Answer from the drawing. Dimensions are ordinates in mm from the lowest x, y and z of the part. A direction names the side the tool comes from. Round coordinates to 2 decimals unless told otherwise and drop trailing zeros. Order: outer loops, then holes, each group sorted by start corner. A loop starts at its lowest first (then second) coordinate and runs counter-clockwise, first axis right, second up. Notation, with made-up numbers: (31.25, 33) -> (35.25, 33) arc R17 cw to (35.25, 64) -> close; hole circle Ø5 at (41, -38). An arc over 180 degrees is marked (long way). Use a Markdown table: item, result. Add a question column.
1. Section C-C, the plane x = 6 is taken. Give the vertices of the cut face in (y, z).
2. Section D-D, the plane y = 13 is taken. Give the vertices of the cut face in (x, z).
3. Section B-B, the plane y = 22 is taken. Give the vertices of the cut face in (x, z).
4. Given pin 1 (12 mm diameter, centred on x = 29.5, y = 14.5, fed in from +Z); pin 2 (9 mm diameter, centred on x = 30, y = 22, fed in from +Z); pin 3 (1.5 mm diameter, centred on x = 34, z = 25.5, fed in from +Y), each flat-ended and moving along its own axis, determine where each tip first touches the part or whether it passes through.
5. For the marked faces 1 and 2, determine the directions among +Z, -Z, +X, -X, +Y, -Y from which every point of the face is accessible in a straight line to the end or side of a thin tool.
6. Section A-A, the plane x = 26 is taken. Give the vertices of the cut face in (y, z).
7. Consider L1, parallel to Y at x = 40, z = 1.1; L2, parallel to Y at x = 16, z = 2.15; L3, parallel to Y at x = 20, z = 15. Determine where each line is inside the solid, lowest interval first. Write a range as [from, to].
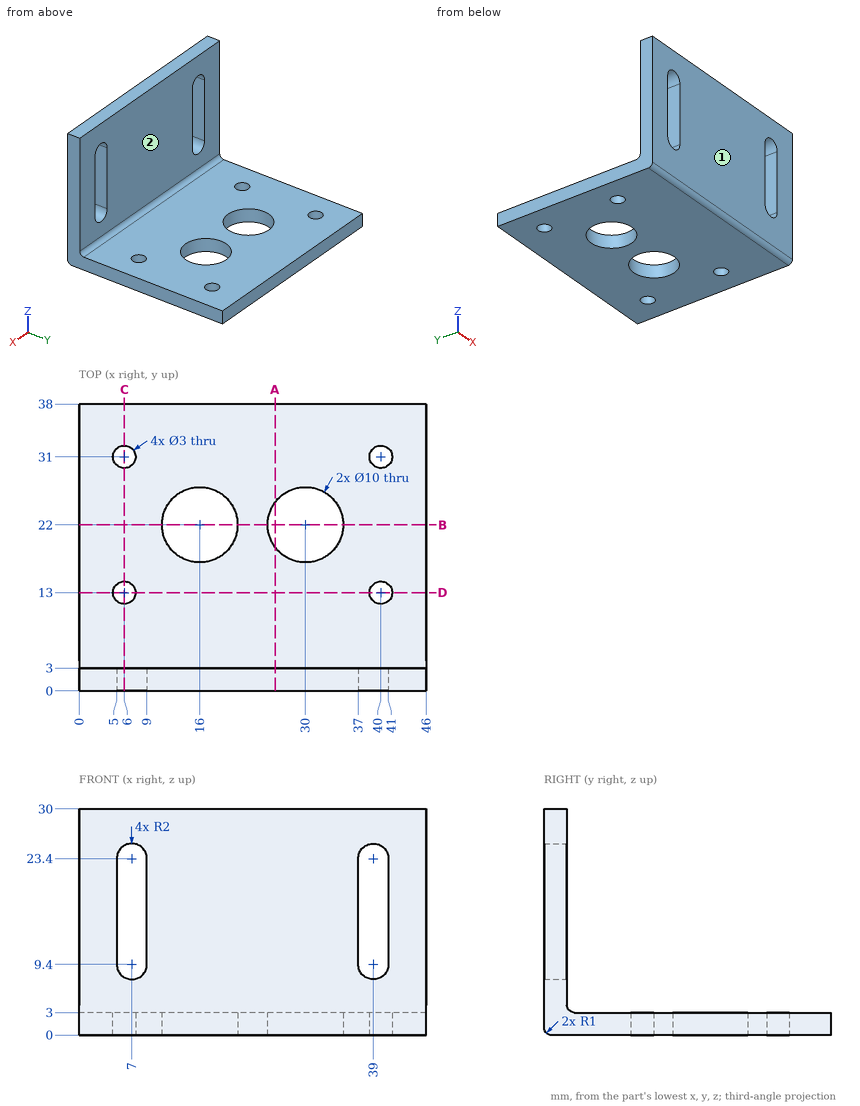
Verdict:
| question | item | result |
|---|---|---|
| 1 | outline | (0, 1) arc R1 ccw to (1, 0) -> (11.5, 0) -> (11.5, 3) -> (4, 3) arc R1 cw to (3, 4) -> (3, 7.67) -> (0, 7.67) -> close; (0, 25.13) -> (3, 25.13) -> (3, 30) -> (0, 30) -> close; (14.5, 0) -> (29.5, 0) -> (29.5, 3) -> (14.5, 3) -> close; (32.5, 0) -> (38, 0) -> (38, 3) -> (32.5, 3) -> close |
| 2 | outline | (0, 0) -> (4.5, 0) -> (4.5, 3) -> (0, 3) -> close; (7.5, 0) -> (38.5, 0) -> (38.5, 3) -> (7.5, 3) -> close; (41.5, 0) -> (46, 0) -> (46, 3) -> (41.5, 3) -> close |
| 3 | outline | (0, 0) -> (11, 0) -> (11, 3) -> (0, 3) -> close; (21, 0) -> (25, 0) -> (25, 3) -> (21, 3) -> close; (35, 0) -> (46, 0) -> (46, 3) -> (35, 3) -> close |
| 4 | pin 1 | stops at z = 3 |
| 4 | pin 2 | passes through |
| 4 | pin 3 | stops at y = 3 |
| 5 | face 1 | +Z, -Z, +X, -X, -Y |
| 5 | face 2 | +Z, +X, -X, +Y |
| 6 | outline | (0, 1) arc R1 ccw to (1, 0) -> (19, 0) -> (19, 3) -> (4, 3) arc R1 cw to (3, 4) -> (3, 30) -> (0, 30) -> close; (25, 0) -> (38, 0) -> (38, 3) -> (25, 3) -> close |
| 7 | L1 | y = [0, 11.5], [14.5, 29.5], [32.5, 38] |
| 7 | L2 | y = [0, 17], [27, 38] |
| 7 | L3 | y = [0, 3] |
